Model file for the job. Use its own axes, mm. Coordinates: 2 decimals unless noted, no trailing zeros. Order: outer loops, then holes, each group sorted by start corner. A loop starts at its lowest first (then second) coordinate and runs counter-clockwise, first axis right, second up. Notation, with made-up numbers: (55.5, -5.75) -> (73.5, -5.75) arc R22 ccw to (73.5, 5.25) -> close; hole circle Ø11 at (-32.5, 71.25). An arc over 180 degrees is marked (long way). Return JSON: item names as keys, results as strings. Group by question number.
1) Probe line 1 (Z direction, x = 44.45, y = 0.3); line 2 (X direction, y = 0.75, z = 36); line 3 (X direction, y = 0.15, z = -2). List the from-to ranges inside material, lowest first.
2) Cut at A-A (y = 0.75). Write the cut outline in (x, z) (3 decimals), and give its area (3 significant figures).
3) Pull direction Z, two halves, no side cores. Call faces 1 (the cylindrical face through (25.77, 0.8, -35.48)), 2 (the cylindrical face through (306.06, 0.78, 0.87)), 3 (the flat face through (164, 0, -1)): +Z half, -Z half, draft (parallel to the pull), parting line (faces both ways), or undercut.
4) Cut at B-B (z = -16.5). Write the cut outline in (x, y).
5) Flat gauge pins, fed straight in: pin 1 (2.5 mm diameter, centred on x = 222.25, z = -36.195, fed in from +Y); pin 2 (1.3 mm diameter, centred on x = 222.25, z = 36.195, fed in from +Y) (1 decimal). Where does each tip first touch, or does it go through?
from build123d import *

# Parameters (mm, degrees)
SKETCH1_R           = 1.0922
BOSS_EXTRUDE1_DEPTH = 1.5875
FILLET1_R           = 6.35


with BuildPart() as part:
    # Sketch1 → Boss-Extrude1 (new body)
    with BuildSketch(Plane(origin=(0, 0, 0), x_dir=(1, 0, 0), z_dir=(0, 1, 0))):
        with BuildLine():
            Line((266.7, 39.37), (0, 39.37))
            ThreePointArc((0, 39.37), (39.37, 0), (0, -39.37))
            Line((0, -39.37), (266.7, -39.37))
            ThreePointArc((266.7, -39.37), (306.07, 0), (266.7, 39.37))
        make_face()
        with Locations((302.895, 0)):
            Circle(SKETCH1_R, mode=Mode.SUBTRACT)
        with Locations((222.25, 36.195)):
            Circle(SKETCH1_R, mode=Mode.SUBTRACT)
        with Locations((44.45, 36.195)):
            Circle(SKETCH1_R, mode=Mode.SUBTRACT)
        with Locations((44.45, -36.195)):
            Circle(SKETCH1_R, mode=Mode.SUBTRACT)
        with Locations((222.25, -36.195)):
            Circle(SKETCH1_R, mode=Mode.SUBTRACT)
    extrude(amount=BOSS_EXTRUDE1_DEPTH)

    # Fillet1
    fillet1_edges = [part.edges().sort_by_distance(p)[0] for p in [
        (0, 0.79375, 39.37),
        (0, 0.79375, -39.37),
    ]]
    fillet(fillet1_edges, radius=FILLET1_R)


solid = part.part
Answers below:
{
 "1": {"line 1": "z = -39.37 to -37.29, -35.1 to 35.1, 37.29 to 39.37", "line 2": "x = 26.02 to 43.38, 45.52 to 221.18, 223.32 to 282.64", "line 3": "x = 39.32 to 306.02"},
 "2": {"outline": "(27.231, -28.434) arc R6.35 ccw to (31.623, -39.37) -> (266.7, -39.37) arc R39.37 ccw to (266.7, 39.37) -> (31.623, 39.37) arc R6.35 ccw to (27.231, 28.434) arc R39.37 cw to start; hole circle Ø2.184 at (44.45, -36.195); hole circle Ø2.184 at (44.45, 36.195); hole circle Ø2.184 at (222.25, -36.195); hole circle Ø2.184 at (222.25, 36.195); hole circle Ø2.184 at (302.895, 0)", "area": "20,800 mm^2"},
 "3": {"face 1": "undercut", "face 2": "parting line", "face 3": "draft"},
 "4": {"outline": "(35.75, 0) -> (302.45, 0) -> (302.45, 1.59) -> (35.75, 1.59) -> close"},
 "5": {"pin 1": "stops at y = 1.59", "pin 2": "passes through"}
}
